Build history of the part. All positions in model axes, mm. A direction names the side the tool comes from. Round coordinates to 2 decimals unless told otherwise and drop trailing zeros. Write each loop counter-clockwise with the first axis right and the second up, starting at its lowest first coordinate (ties: lowest second). Pieces come first, ordered by that corner, then holes. Notation, with made-up numbers: (30.25, -29.5) -> (84.25, -29.5) arc R23 cw to (84.25, -15.5) -> close; hole circle Ø5 at (51.25, 72.25). An arc over 180 degrees is marked (long way). Answer in a Markdown table with one row per item.
Autodesk Inventor part; units mm, degrees
ref_plane "YZ Plane" through (0, 0, 0) normal (1, 0, 0) x (0, 1, 0)
ref_plane "XZ Plane" through (0, 0, 0) normal (0, 1, 0) x (-1, 0, 0)
ref_plane "XY Plane" through (0, 0, 0) normal (0, 0, 1) x (1, 0, 0)
ref_plane "Work Plane1" through (0, 0, 0) normal (0, 0, 1) x (1, 0, 0)
sketch "Sketch1" plane through (0, 0, 0) normal (0, 0, 1) x (1, 0, 0)
  line L0 (254.7, 154.94) -> (254.7, 140.97)
  line L1 (254.7, -154.94) -> (254.7, 140.97)
  arc A0 (254.7, 154.94) -> (250.89, 158.75) centre (250.89, 154.94) ccw
  line L2 (-274.89, 158.75) -> (250.89, 158.75)
  arc A1 (260.25, -24.13) -> (261.52, -25.4) centre (261.52, -24.13) ccw
  line L3 (260.25, -24.13) -> (260.25, -21.59)
  arc A2 (261.52, -20.32) -> (260.25, -21.59) centre (261.52, -21.59) ccw
  line L4 (261.52, -20.32) -> (265.66, -20.32)
  arc A3 (266.93, -21.59) -> (265.66, -20.32) centre (265.66, -21.59) ccw
  line L5 (266.93, -21.59) -> (266.93, -24.13)
  arc A4 (265.66, -25.4) -> (266.93, -24.13) centre (265.66, -24.13) ccw
  line L6 (265.66, -25.4) -> (261.52, -25.4)
  arc A5 (-288.0375, 171.2625) -> (-291.2125, 168.0875) centre (-288.0375, 168.0875) ccw
  line L7 (-291.2125, -168.0875) -> (-291.2125, 168.0875)
  arc A6 (-291.2125, -168.0875) -> (-288.0375, -171.2625) centre (-288.0375, -168.0875) ccw
  line L8 (288.0375, -171.2625) -> (-288.0375, -171.2625)
  arc A7 (288.0375, -171.2625) -> (291.2125, -168.0875) centre (288.0375, -168.0875) ccw
  line L9 (291.2125, 168.0875) -> (291.2125, -168.0875)
  arc A8 (291.2125, 168.0875) -> (288.0375, 171.2625) centre (288.0375, 168.0875) ccw
  line L10 (-288.0375, 171.2625) -> (288.0375, 171.2625)
  circle A9 centre (264.3, 19.25) radius 3.6
  line L11 (295.2621, 171.2883) -> (295.2621, 171.2625)
  line L12 (291.2125, 120.65) -> (254.7, 120.65)
  line L13 (215.0125, 171.2625) -> (215.0125, 158.75)
  point P0 (0, 0)
extrude "Extrusion1" add sketch "Sketch1" along normal blind 25.4 contours A0 L2 L13 L10 A8 L9 L12 L1 L0
chamfer "Chamfer1" distance 3.175 angle 45 3 edges at (254.7, 130.81, 25.4) (253.5841, 157.6341, 25.4) (232.9512, 158.75, 25.4)
properties material "ABS Plastic"
Q1. Drop a flat-ended pin along its axis: P1, Ø11, axis at y = 141.5, z = 10.5, coming from the -X side. Give the stop position or say it passes through.
A:
| item | result |
|---|---|
| P1 | x = 254.7 |
Q2. Saw through at A-A on y = 132.5. Write the cut outline in (x, z) (1 decimal).
A:
| item | result |
|---|---|
| outline | (254.7, 0) -> (291.2, 0) -> (291.2, 25.4) -> (257.9, 25.4) -> (254.7, 22.2) -> close |
Q3. Which spindle directions (+Z, -Z, +X, -X, +Y, -Y) get a long thin tool onto all of the face, cutting with end or side? Do faces 1 (the flat face through (233, 158.75, 11)), 2 (the flat face through (256.31, 137.555, 23.835)), 3 (the cylindrical face through (290.258, 170.357, 12.522)). Say none if no direction does.
A:
| item | result |
|---|---|
| face 1 | +Z, -Z, -X, -Y |
| face 2 | +Z, -X, -Y |
| face 3 | +Z, -Z, +X, +Y |
Q4. Wall check: line 1 (Y direction, x = 237, z = 5.75); line 2 (X direction, y = 131.5, z = 6.25); line 3 (Z direction, x = 228.5, y = 160) (3 decimals). Give the ranges that are in metal, low to high. Write a range as [from, to].
A:
| item | result |
|---|---|
| line 1 | [158.75, 171.26] |
| line 2 | [254.7, 291.21] |
| line 3 | [0, 23.475] |
